Work out the finished part from the listing and answer in its coordinate system (mm). A direction names the side the tool comes from. Round coordinates to 2 decimals unless told otherwise and drop trailing zeros. Loops run counter-clockwise (first coordinate to the right, second up) from the corner with the lowest first, then second, coordinate; pieces in that order, holes last. Notation, with made-up numbers: (21, 48) - (39, 48) arc R18 ccw to (39, 83) - close; hole circle Ø5 at (-17, -33.75). An arc over 180 degrees is marked (long way). Answer as CSV lines item,"result". Start each with the question number.
Q1. The mould has two halves that part along X. Classify faces 3 (the face through (12.79, 15.24, 3.22)), 4 (the face through (15, 6, 0)), 5 (the face through (17.147, 1.932, -3.259)): +X half, -X half, draft (parallel to the pull), parting line (faces both ways), or undercut.
Q2. For faces 1 (the face through (13, 4, 6.35)), 2 (the face through (13, 3.81, -3)), determine the directions among +Z, -Z, +X, -X, +Y, -Y from which every point of the face is accessible in a straight line to the end or side of a thin tool.
Q3. Section C-C on z = 1.25 is taken. Write down the section's boundary in (x, y) (3 decimals).
Q4. Each of these flat-tipped pins is pushed along its axis until it touches: pin 1 Ø4 at (x, z) = (20.5, 1.5) entering from +Y; pin 2 Ø7.5 at (x, y) = (12.7, 8.89) entering from -Z; pin 3 Ø1.5 at (x, y) = (15.5, 9) entering from +Z; pin 4 Ø4 at (y, z) = (4, -4) entering from +X. Where does it stop, or does it pass through?
Q5. Section D-D on y = 8 is taken. Write down the section's boundary in (x, z).
Q6. Straight lines are drawn through the part: L1, parallel to Y at x = 12.7, z = 5.25 (3 decimals); L2, parallel to Z at x = 19.05, y = 1.35; L3, parallel to X at y = 2.75, z = -3.75. For each, find the intervals that lie inside material, in ascending order. Write a range as [from, to].
Q7. Section A-A on x = 12.7 is taken. Write down the section's boundary in (y, z) (3 decimals).
Q8. Section B-B on y = 10.75 is taken. Write down the section's boundary in (x, z), then the cut area to 3 significant figures.
```python
from build123d import *

# Parameters (mm, degrees)
SKETCH2_R           = 3.175
BOSS_EXTRUDE2_DEPTH = 6.35
SKETCH6_W           = 20.852651852
SKETCH6_H           = 11.43
CUT_EXTRUDE3_DEPTH  = 6.35
SKETCH7_R           = 1.905
CUT_EXTRUDE4_DEPTH  = 6.35


with BuildPart() as part:
    # Sketch2 → Boss-Extrude2 (new body, symmetric)
    with BuildSketch(Plane.XY):
        with BuildLine():
            Line((0, 0), (25.4, 0))
            Line((25.4, 0), (18.152847328, 12.144067611))
            ThreePointArc((18.152847328, 12.144067611), (12.7, 15.24), (7.247152672, 12.144067611))
            Line((7.247152672, 12.144067611), (0, 0))
        make_face()
        with Locations((12.7, 8.89)):
            Circle(SKETCH2_R, mode=Mode.SUBTRACT)
    extrude(amount=BOSS_EXTRUDE2_DEPTH, both=True)

    # Sketch6 → Cut-Extrude3 (cut)
    with BuildSketch(Plane.XY):
        with Locations((12.7, 9.525)):
            Rectangle(SKETCH6_W, SKETCH6_H)
    extrude(amount=-CUT_EXTRUDE3_DEPTH, mode=Mode.SUBTRACT)

    # Sketch7 → Cut-Extrude4 (cut)
    with BuildSketch(Plane(origin=(0, 3.81, 0), x_dir=(1, 0, 0), z_dir=(0, 1, 0))):
        with Locations((6.35, 3.175)):
            Circle(SKETCH7_R)
        with Locations((19.05, 3.175)):
            Circle(SKETCH7_R)
    extrude(amount=-CUT_EXTRUDE4_DEPTH, mode=Mode.SUBTRACT)


solid = part.part
```
Findings:
1,face 3,"parting line"
1,face 4,"draft"
1,face 5,"undercut"
2,face 1,"+Z, +X, -X, +Y, -Y"
2,face 2,"-Z, +X, -X, +Y"
3,outline,"(0, 0) - (25.4, 0) - (18.153, 12.144) arc R6.35 ccw to (7.247, 12.144) - close; hole circle Ø6.35 at (12.7, 8.89)"
4,pin 1,"stops at y = 11.56"
4,pin 2,"stops at z = 0"
4,pin 3,"stops at z = 6.35"
4,pin 4,"stops at x = 24.21"
5,outline,"(4.77, 0) - (9.65, 0) - (9.65, 6.35) - (4.77, 6.35) - close; (15.75, 0) - (20.63, 0) - (20.63, 6.35) - (15.75, 6.35) - close"
6,L1,"y = [0, 5.715], [12.065, 15.24]"
6,L2,"z = [-6.35, -5.08], [-1.27, 6.35]"
6,L3,"x = [1.64, 4.53], [8.17, 17.23], [20.87, 23.76]"
7,outline,"(0, -6.35) - (3.81, -6.35) - (3.81, 0) - (5.715, 0) - (5.715, 6.35) - (0, 6.35) - close; (12.065, 0) - (15.24, 0) - (15.24, 6.35) - (12.065, 6.35) - close"
8,outline,"(6.42, 0) - (10.13, 0) - (10.13, 6.35) - (6.42, 6.35) - close; (15.27, 0) - (18.98, 0) - (18.98, 6.35) - (15.27, 6.35) - close"
8,area,"47.1 mm^2"
